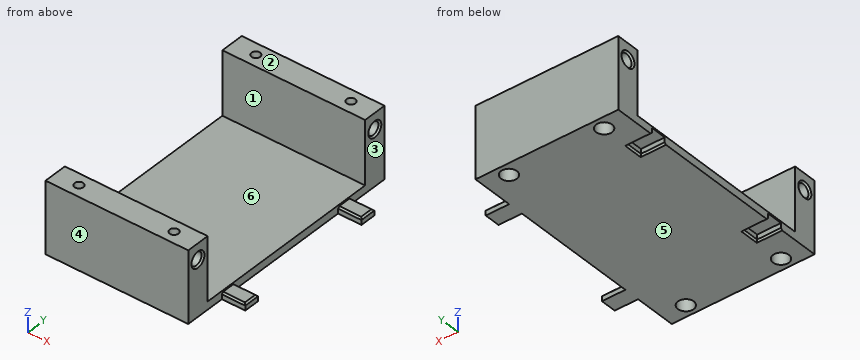
```python
from build123d import *

# Parameters (mm, degrees)
SKETCH_W        = 90
SKETCH_H        = 152
PAD_DEPTH       = 5
SKETCH001_W     = 14.75
SKETCH001_H     = 9.9
PAD001_DEPTH    = 4
SKETCH002_W     = 15
SKETCH002_H     = 10
POCKET_DEPTH    = 4
SKETCH003_W     = 90
SKETCH003_H     = 15
PAD002_DEPTH    = 40
SKETCH004_R     = 2.75
POCKET001_DEPTH = 45.001
SKETCH005_R     = 5
POCKET002_DEPTH = 34
CHAMFER_SIZE    = 1
SKETCH006_R     = 4.05
POCKET003_DEPTH = 9
SKETCH007_R     = 4.05
POCKET004_DEPTH = 9
CHAMFER001_SIZE = 1


with BuildPart() as part:
    # Sketch → Pad (new body)
    with BuildSketch(Plane.XY):
        with Locations((45, 76)):
            Rectangle(SKETCH_W, SKETCH_H)
    extrude(amount=PAD_DEPTH)

    # Sketch001 (on Face5 of Pad) → Pad001 (join)
    with BuildSketch(Plane(origin=(0, 0, 0), x_dir=(1, 0, 0), z_dir=(0, 0, -1))):
        with Locations((97.375, -31)):
            Rectangle(SKETCH001_W, SKETCH001_H)
        with Locations((97.375, -121)):
            Rectangle(SKETCH001_W, SKETCH001_H)
    extrude(amount=-PAD001_DEPTH)

    # Sketch002 (on Face14 of Pad001) → Pocket (cut)
    with BuildSketch(Plane(origin=(0, 0, 0), x_dir=(1, 0, 0), z_dir=(0, 0, -1))):
        with Locations((7.5, -31)):
            Rectangle(SKETCH002_W, SKETCH002_H)
        with Locations((7.5, -121)):
            Rectangle(SKETCH002_W, SKETCH002_H)
    extrude(amount=-POCKET_DEPTH, mode=Mode.SUBTRACT)

    # Sketch003 (on Face5 of Pocket) → Pad002 (join)
    with BuildSketch(Plane.XY.offset(5)):
        with Locations((45, 144.5)):
            Rectangle(SKETCH003_W, SKETCH003_H)
        with Locations((45, 7.5)):
            Rectangle(SKETCH003_W, SKETCH003_H)
    extrude(amount=PAD002_DEPTH)

    # Sketch004 (on Face1 of Pad002) → Pocket001 (cut, through all)
    with BuildSketch(Plane(origin=(0, 0, 0), x_dir=(1, 0, 0), z_dir=(0, 0, -1))):
        with Locations((15, -7.5)):
            Circle(SKETCH004_R)
        with Locations((75, -7.5)):
            Circle(SKETCH004_R)
        with Locations((75, -144.5)):
            Circle(SKETCH004_R)
        with Locations((15, -144.5)):
            Circle(SKETCH004_R)
    extrude(amount=-POCKET001_DEPTH, mode=Mode.SUBTRACT)

    # Sketch005 (on Face1 of Pocket001) → Pocket002 (cut)
    with BuildSketch(Plane(origin=(0, 0, 0), x_dir=(1, 0, 0), z_dir=(0, 0, -1))):
        with Locations((15, -7.5)):
            Circle(SKETCH005_R)
        with Locations((75, -7.5)):
            Circle(SKETCH005_R)
        with Locations((75, -144.5)):
            Circle(SKETCH005_R)
        with Locations((15, -144.5)):
            Circle(SKETCH005_R)
    extrude(amount=-POCKET002_DEPTH, mode=Mode.SUBTRACT)

    # Chamfer
    chamfer_edges = [part.edges().sort_by_distance(p)[0] for p in [
        (97.375, 116.05, 4),
        (104.75, 121, 4),
        (97.375, 125.95, 4),
        (104.75, 31, 4),
        (97.375, 35.95, 4),
        (97.375, 26.05, 4),
        (7.5, 36, 0),
        (15, 31, 0),
        (7.5, 26, 0),
        (7.5, 126, 0),
        (15, 121, 0),
        (7.5, 116, 0),
    ]]
    chamfer(chamfer_edges, length=CHAMFER_SIZE)

    # Sketch006 (on Face6 of Chamfer) → Pocket003 (cut)
    with BuildSketch(Plane.YZ.offset(90)):
        with Locations((7.5, 35)):
            Circle(SKETCH006_R)
        with Locations((144.5, 35)):
            Circle(SKETCH006_R)
    extrude(amount=-POCKET003_DEPTH, mode=Mode.SUBTRACT)

    # Sketch007 (on Face2 of Pocket003) → Pocket004 (cut)
    with BuildSketch(Plane(origin=(0, 0, 0), x_dir=(0, -1, 0), z_dir=(-1, 0, 0))):
        with Locations((-144.5, 35)):
            Circle(SKETCH007_R)
        with Locations((-7.5, 35)):
            Circle(SKETCH007_R)
    extrude(amount=-POCKET004_DEPTH, mode=Mode.SUBTRACT)

    # Chamfer001
    chamfer001_edges = [part.edges().sort_by_distance(p)[0] for p in [
        (0, 11.55, 35),
        (0, 148.55, 35),
        (90, 3.45, 35),
        (90, 140.45, 35),
    ]]
    chamfer(chamfer001_edges, length=CHAMFER001_SIZE)


solid = part.part
```
The model under review builds one solid part; all positions refer to its coordinate system, in mm. Face numbers are marked on the shaded views. A direction names the side the tool comes from. Round coordinates to 2 decimals unless told otherwise and drop trailing zeros. Loops run counter-clockwise (first coordinate to the right, second up) from the corner with the lowest first, then second, coordinate; pieces in that order, holes last. Notation, with made-up numbers: M 77.25,-6 L 99.25,-6 A24 ccw 99.25,26 Z; hole C 37,4.25 d8. An arc over 180 degrees is marked long. Put each result on its own line as item: value.
Q1. Consider section B-B, the plane y = 7.5. Count the separate pieces of the cut face and the enclosed holes in it, then the cut area to 3 significant figures.
Result set:
separate pieces: 3
enclosed holes: 0
area: 3,100 mm²
Q2. Consider section A-A, the plane z = 11. Give the boundary of the cut face in (x, y), then the cut area to 3 significant figures.
Result set:
outline: M 0,0 L 90,0 L 90,15 L 0,15 Z; M 0,137 L 90,137 L 90,152 L 0,152 Z; hole C 15,7.5 d10; hole C 15,144.5 d10; hole C 75,7.5 d10; hole C 75,144.5 d10
area: 2,390 mm²
Q3. Consider section C-C, the plane x = 75. Give the boundary of the cut face in (y, z).
Result set:
outline: M 0,0 L 2.5,0 L 2.5,34 L 4.75,34 L 4.75,45 L 0,45 Z; M 10.25,34 L 12.5,34 L 12.5,0 L 139.5,0 L 139.5,34 L 141.75,34 L 141.75,45 L 137,45 L 137,5 L 15,5 L 15,45 L 10.25,45 Z; M 147.25,34 L 149.5,34 L 149.5,0 L 152,0 L 152,45 L 147.25,45 Z
Q4. Consider section D-D, the plane x = 49. Give the boundary of the cut face in (y, z), then the cut area to 3 significant figures.
Result set:
outline: M 0,0 L 152,0 L 152,45 L 137,45 L 137,5 L 15,5 L 15,45 L 0,45 Z
area: 1,960 mm²
Q5. To check wall thickness, follow L1, parallel to X at y = 144, z = 25; L2, parallel to Z at x = 6.5, y = 7.5; L3, parallel to X at y = 7.5, z = 40.5. State the ranges of each line that lie inside material, in increasing order.
Result set:
L1: x = 0 to 10.03, 19.97 to 70.03, 79.97 to 90
L2: z = 0 to 30.95, 39.05 to 45
L3: x = 0 to 12.25, 17.75 to 72.25, 77.75 to 90
Q6. Mouldability with a two-part tool opening along Y and no side actions: class the marked faces 1, 2, 3 and 4 as released by +Y, released by -Y, zero draft, split by the parting line, or undercut.
Result set:
face 1: undercut
face 2: zero draft
face 3: undercut
face 4: released by -Y
Q7. For pin 1 (0.9 mm diameter, centred on x = 95.5, z = 1.5, fed in from -Y); pin 2 (7.5 mm diameter, centred on y = 7.5, z = 35, fed in from +X); pin 3 (2.5 mm diameter, centred on y = 9.5, z = 36.5, fed in from -X), all flat-tipped, find the tip position at first contact; note any pin that passes through.
Result set:
pin 1: stops at y = 26.05
pin 2: stops at x = 81
pin 3: stops at x = 9
Q8. Machinability: for the marked faces 5 and 6, which of the approach directions +Z, -Z, +X, -X, +Y, -Y give a long, thin tool a straight path to every point of the face, cutting with its end or side? Answer none if there is none.
Result set:
face 5: -Z, +X, -X, +Y, -Y
face 6: +Z, +X, -X
